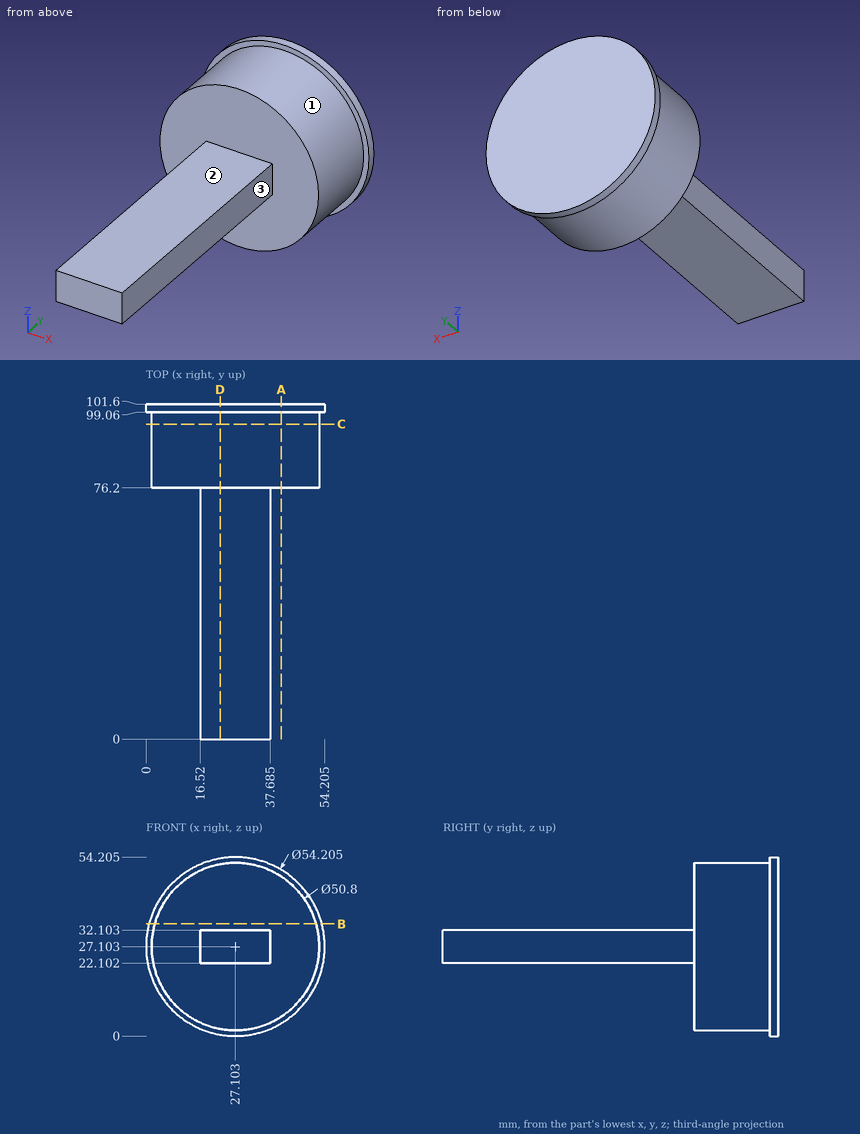
Study the drawing (mm; zero at the part's minimum x, y, z) and answer. A direction names the side the tool comes from. Round coordinates to 2 decimals unless told otherwise and drop trailing zeros. Order: outer loops, then holes, each group sorted by start corner. A loop starts at its lowest first (then second) coordinate and runs counter-clockwise, first axis right, second up. Notation, with made-up numbers: (-38.75, 7.5) - (11.25, 7.5) arc R12 cw to (11.25, 16.5) - close; hole circle Ø10 at (-16.75, 47.25). An arc over 180 degrees is marked (long way). Use one line per item in the form item = value. Start each with the question number.
(1) The part is cut by section A-A (x = 41). Give the vertices of the cut face in (y, z) (1 decimal), then the cut area to 3 significant figures.
(2) The part is cut by section B-B (z = 34). Give the vertices of the cut face in (x, y), then the cut area to 3 significant figures.
(3) The part is cut by section C-C (y = 95.5). Give the vertices of the cut face in (x, z), then the cut area to 3 significant figures.
(4) The part is cut by section D-D (x = 22.5). Give the vertices of the cut face in (y, z), then the cut area to 3 significant figures.
(5) Find the intervals of material crossed by line 1 along Y through (x, z) = (47, 14.5); line 2 along Z through (x, y) = (37, 68); line 3 along X through (y, z) = (26.5, 28.5) (1 decimal), in increasing order. Write a range as from..to.
(6) Flat-ended cylindrical pins translate along their axes: pin 1 Ø8 at (y, z) = (33.5, 26.5) entering from -X; pin 2 Ø6 at (x, y) = (18, 46) entering from -Z; pin 3 Ø11 at (y, z) = (41, 29) entering from +X (1 decimal). Find the tip coordinate at first contact, or state that the pin passes through.
(7) For the marked faces 1, 2 and 3, determine the directions among +Z, -Z, +X, -X, +Y, -Y from which every point of the face is accessible in a straight line to the end or side of a thin tool.
Checked values:
q1.outline = (76.2, 5.8) - (99.1, 5.8) - (99.1, 3.8) - (101.6, 3.8) - (101.6, 50.4) - (99.1, 50.4) - (99.1, 48.4) - (76.2, 48.4) - close
q1.area = 1,090 mm^2
q2.outline = (0.89, 99.06) - (2.66, 99.06) - (2.66, 76.2) - (51.55, 76.2) - (51.55, 99.06) - (53.31, 99.06) - (53.31, 101.6) - (0.89, 101.6) - close
q2.area = 1,250 mm^2
q3.outline = circle Ø50.8 at (27.1, 27.1)
q3.area = 2,030 mm^2
q4.outline = (0, 22.1) - (76.2, 22.1) - (76.2, 2.12) - (99.06, 2.12) - (99.06, 0.39) - (101.6, 0.39) - (101.6, 53.81) - (99.06, 53.81) - (99.06, 52.08) - (76.2, 52.08) - (76.2, 32.1) - (0, 32.1) - close
q4.area = 2,040 mm^2
q5.line_1 = 76.2..101.6
q5.line_2 = 22.1..32.1
q5.line_3 = 16.5..37.7
q6.pin_1 = 16.52
q6.pin_2 = 22.1
q6.pin_3 = 37.7
q7.face_1 = -Y
q7.face_2 = +Z, +X, -X, -Y
q7.face_3 = +Z, -Z, +X, -Y
